```python
from build123d import *

# Parameters (mm, degrees)
SKETCH1_W           = 75
SKETCH1_H           = 30
BOSS_EXTRUDE1_DEPTH = 30
SKETCH3_R           = 5
CUT_EXTRUDE1_DEPTH  = 60
SKETCH4_W           = 1.254965376
SKETCH4_H           = 1
CUT_EXTRUDE2_DEPTH  = 83.158383626
SKETCH5_R           = 2.5
SKETCH5_R_2         = 2.597055459
CUT_EXTRUDE3_DEPTH  = 20
BOSS_EXTRUDE2_START = 5
SKETCH6_R           = 3.75
SKETCH6_R_2         = 2.597055459
SKETCH6_R_3         = 2.5
BOSS_EXTRUDE2_DEPTH = 5
SKETCH7_R           = 2.5
CUT_EXTRUDE4_DEPTH  = 10
SKETCH8_R           = 4.5
SKETCH8_R_2         = 3.5
BOSS_EXTRUDE3_DEPTH = 10
SKETCH9_R           = 1
CUT_EXTRUDE5_DEPTH  = 60.634302243
FILLET1_R           = 10


with BuildPart() as part:
    # Sketch1 → Boss-Extrude1 (new body)
    with BuildSketch(Plane(origin=(0, 0, 0), x_dir=(0, 0, -1), z_dir=(1, 0, 0))):
        Rectangle(SKETCH1_W, SKETCH1_H)
    extrude(amount=BOSS_EXTRUDE1_DEPTH)

    # Sketch3 → Cut-Extrude1 (cut)
    with BuildSketch(Plane(origin=(0, 0, -37.5), x_dir=(-1, 0, 0), z_dir=(0, 0, -1))):
        with Locations((-15, 0)):
            Circle(SKETCH3_R)
    extrude(amount=-CUT_EXTRUDE1_DEPTH, mode=Mode.SUBTRACT)

    # Sketch4 → Cut-Extrude2 (cut, through all)
    with BuildSketch(Plane(origin=(0, 0, -37.5), x_dir=(-1, 0, 0), z_dir=(0, 0, -1))):
        with Locations((-29.372517312, 6.5)):
            Rectangle(SKETCH4_W, SKETCH4_H)
        with Locations((-29.372517312, -6.5)):
            Rectangle(SKETCH4_W, SKETCH4_H)
        with Locations((-0.627482688, -6.5)):
            Rectangle(SKETCH4_W, SKETCH4_H)
        with Locations((-0.627482688, 6.5)):
            Rectangle(SKETCH4_W, SKETCH4_H)
    extrude(amount=-CUT_EXTRUDE2_DEPTH, mode=Mode.SUBTRACT)

    # Sketch5 → Cut-Extrude3 (cut)
    with BuildSketch(Plane(origin=(0, 15, 0), x_dir=(1, 0, 0), z_dir=(0, 1, 0))):
        with Locations(Location((15, 27.5, 0), (0, 0, 270))):
            Circle(SKETCH5_R)
        with Locations(Location((15, -27.5, 0), (0, 0, 270))):
            Circle(SKETCH5_R_2)
    extrude(amount=-CUT_EXTRUDE3_DEPTH, mode=Mode.SUBTRACT)

    # Sketch6 → Boss-Extrude2 (add)
    # profile 1 of 2: a face of its own
    with BuildSketch(Plane(origin=(0, 15, 0), x_dir=(1, 0, 0), z_dir=(0, 1, 0)).offset(BOSS_EXTRUDE2_START)):
        with Locations(Location((15, -27.5, 0), (0, 0, 90))):
            Circle(SKETCH6_R)
        with Locations(Location((15, -27.5, 0), (0, 0, 270))):
            Circle(SKETCH6_R_2, mode=Mode.SUBTRACT)
    # profile 2 of 2: a face of its own
    with BuildSketch(Plane(origin=(0, 15, 0), x_dir=(1, 0, 0), z_dir=(0, 1, 0)).offset(BOSS_EXTRUDE2_START)):
        with Locations(Location((15, 27.5, 0), (0, 0, 90))):
            Circle(SKETCH6_R)
        with Locations(Location((15, 27.5, 0), (0, 0, 270))):
            Circle(SKETCH6_R_3, mode=Mode.SUBTRACT)
    extrude(amount=-BOSS_EXTRUDE2_DEPTH)

    # Sketch7 → Cut-Extrude4 (cut)
    with BuildSketch(Plane(origin=(0, 0, 22.5), x_dir=(-1, 0, 0), z_dir=(0, 0, -1))):
        with Locations((-15, 0)):
            Circle(SKETCH7_R)
    extrude(amount=-CUT_EXTRUDE4_DEPTH, mode=Mode.SUBTRACT)

    # Sketch8 → Boss-Extrude3 (add)
    with BuildSketch(Plane.XY.offset(37.5)):
        with Locations(Location((15, 0, 0), (0, 0, 180))):
            Circle(SKETCH8_R)
        with Locations((15, 0)):
            Circle(SKETCH8_R_2, mode=Mode.SUBTRACT)
    extrude(amount=BOSS_EXTRUDE3_DEPTH)

    # Sketch9 → Cut-Extrude5 (cut, through all)
    with BuildSketch(Plane(origin=(0, 0, 0), x_dir=(0, 0, -1), z_dir=(1, 0, 0))):
        with Locations(Location((-42.457775401, 0, 0), (0, 0, 180))):
            Circle(SKETCH9_R)
    extrude(amount=CUT_EXTRUDE5_DEPTH, mode=Mode.SUBTRACT)

    # Fillet1
    # the kernel refuses this fillet: 10 mm, written as the material it takes off along each edge
    with BuildSketch(Plane(origin=(30, -15, 61.994897428), x_dir=(-1, 0, 0), z_dir=(0, 0, -1)), Plane(origin=(30, 15, -61.994897428), x_dir=(-1, 0, 0), z_dir=(0, 0, 1))) as fillet1_piece_1:
        with BuildLine():
            CenterArc((9.797958971, 10), FILLET1_R, 191.536959033, 78.463040967)
            Line((0, 8), (-0.195959179, 7.96))
            ThreePointArc((-0.195959179, 7.96), (-0.2, 4), (-0.2, 0))
            Line((-0.2, 0), (0, -0.2))
            Line((0, -0.2), (9.797958971, -0.2))
            Line((9.797958971, -0.2), (9.797958971, 0))
        make_face()
    extrude(amount=123.989794856, mode=Mode.SUBTRACT)
    with BuildSketch(Plane(origin=(0, -15, 61.994897428), x_dir=(1, 0, 0), z_dir=(0, 0, -1))) as fillet1_piece_2:
        with BuildLine():
            CenterArc((9.797958971, -10), FILLET1_R, 90, 78.463040967)
            Line((0, -8), (-0.195959179, -7.96))
            ThreePointArc((-0.195959179, -7.96), (-0.2, -4), (-0.2, 0))
            Line((-0.2, 0), (0, 0.2))
            Line((0, 0.2), (9.797958971, 0.2))
            Line((9.797958971, 0.2), (9.797958971, 0))
        make_face()
    extrude(amount=123.989794856, mode=Mode.SUBTRACT)
    with BuildSketch(Plane(origin=(0, 15, -61.994897428), x_dir=(0, -1, 0), z_dir=(0, 0, 1))) as fillet1_piece_3:
        with BuildLine():
            CenterArc((10, 9.797958971), FILLET1_R, 180, 78.463040967)
            Line((0, 9.797958971), (-0.2, 9.797958971))
            Line((-0.2, 9.797958971), (-0.2, 0))
            Line((-0.2, 0), (0, -0.2))
            ThreePointArc((0, -0.2), (4, -0.2), (7.96, -0.195959179))
            Line((7.96, -0.195959179), (8, 0))
        make_face()
    extrude(amount=123.989794856, mode=Mode.SUBTRACT)


solid = part.part
```
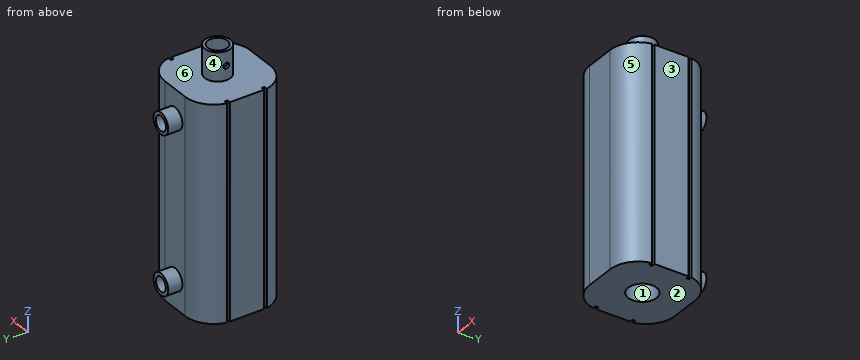
Could you check a few things on this model? Use its own coordinates, in mm. Face numbers are marked on the shaded views. A direction names the side the tool comes from. Round coordinates to 2 decimals unless told otherwise and drop trailing zeros. Loops run counter-clockwise (first coordinate to the right, second up) from the corner with the lowest first, then second, coordinate; pieces in that order, holes last. Notation, with made-up numbers: M 4.25,84.25 L 25.25,84.25 A11 cw 25.25,100.25 Z; hole C 23,-7 d9. An arc over 180 degrees is marked long. Write item = value, one per line.
1. I need wall thicknesses on probe 1 along Z at (x, y) = (15, 9.75); probe 2 along X at (y, z) = (0, 23.55); probe 3 along Z at (x, y) = (16, 14.5). Which ranges of each line are inside material? Lowest first, please.
Results below:
probe_1 = -37.5 to -30, -25 to 24.9, 30.1 to 37.5
probe_2 = 0 to 12.5, 17.5 to 30
probe_3 = -37.5 to -29.79, -25.21 to 25.1, 29.9 to 37.5
2. I want a section at C-C, the plane x = 26. Write out the boundary of the cut face in (y, z).
Results below:
outline = M -13.15,-37.5 L 13.15,-37.5 L 13.15,37.5 L -13.15,37.5 Z
3. Which directions (+Z, -Z, +X, -X, +Y, -Y) give clear straight access to the entire face, cutting with the end or side of a thin tool? Please do the marked faces 5 and 6.
Results below:
face_5 = +Z, -Z, +X, -Y
face_6 = +Z
4. Will these pins go through, and if not, where does the flat tip stop? P1, Ø4.5, axis at x = 15, y = 0, coming from the -Z side; P2, Ø6, axis at x = 15, y = 0, coming from the -Z side; P3, Ø0.6, axis at x = 0.5, z = -12, coming from the +Y side.
Results below:
P1 = 32.5
P2 = 22.5
P3 = 9.36
5. I want a section at D-D, the plane y = -11. Write out the boundary of the cut face in (x, z).
Results below:
outline = M 1.8,-37.5 L 28.2,-37.5 L 28.2,37.5 L 1.8,37.5 Z
6. I want a section at A-A, the plane z = -1. Write out the boundary of the cut face in (x, y), and give its area (3 significant figures).
Results below:
outline = M 0,-7 A10 ccw 9.8,-15 L 20.2,-15 A10 ccw 30,-7 L 28.75,-7 L 28.75,-6 L 30,-6 L 30,6 L 28.75,6 L 28.75,7 L 30,7 A10 ccw 20.2,15 L 9.8,15 A10 ccw 0,7 L 1.25,7 L 1.25,6 L 0,6 L 0,-6 L 1.25,-6 L 1.25,-7 Z; hole C 15,0 d10
area = 738 mm²
7. Thinking about a two-plate mould opening in X: for the marked faces 1, 2, 3 and 4, which applies, +X half, -X half, draft (parallel to the pull), parting line (faces both ways), or undercut?
Results below:
face_1 = undercut
face_2 = draft
face_3 = +X half
face_4 = parting line
